Autodesk Inventor part; units mm, degrees
ref_plane "YZ Plane" through (0, 0, 0) normal (1, 0, 0) x (0, 1, 0)
ref_plane "XZ Plane" through (0, 0, 0) normal (0, 1, 0) x (-1, 0, 0)
ref_plane "XY Plane" through (0, 0, 0) normal (0, 0, 1) x (1, 0, 0)
sketch "Sketch1" plane through (0, 0, 0) normal (1, 0, 0) x (0, 1, 0)
  circle A0 centre (0, 0) radius 70
  line L0 (0, 0) -> (66.7602, 21.0494) construction
  line L1 (66.7602, -21.0494) -> (0, 0) construction
  line L2 (66.7602, -21.0494) -> (66.7602, 21.0494) construction
  circle A1 centre (66.7602, 21.0494) radius 1.65
  circle A2 centre (66.7602, -21.0494) radius 1.65
  circle A3 centre (0, 0) radius 57.5
  line L3 (64.3545, 28.6791) -> (-26.6041, 0)
  line L4 (-26.6041, 0) -> (64.3545, -28.6791)
  line L5 (74.7602, -21.0494) -> (74.7602, 21.0494)
  arc A4 (74.7602, 21.0494) -> (64.3545, 28.6791) centre (66.7602, 21.0494) ccw
  arc A5 (64.3545, -28.6791) -> (74.7602, -21.0494) centre (66.7602, -21.0494) ccw
  circle A6 centre (0, 0) radius 64.5
  point P0 (66.7602, 0)
  point P1 (51.8997, 24.7522)
  point P2 (51.8997, -24.7522)
  point P3 (58.6341, 26.8755)
  point P4 (58.6341, -26.8755)
  dimension "d0" = 140
  dimension "d1" = 35
  dimension "d2" = 3.3
  dimension "d3" = 3.3
  dimension "d4" = 115
  dimension "d5" = 8
  dimension "d6" = 8
  dimension "d7" = 7
extrude "Extrusion1" add sketch "Sketch1" against normal blind 7 contours A0 A2 L4 A6 L3 A1 | A0 A1 L3 A4 L5 A5 L4 A2 | A6 L4 A3 L3 picked at (61.9464, 3.0696)
extrude "Extrusion2" add sketch "Sketch1" along normal blind 20 contours A6 L4 A3 L3 picked at (61.9464, 3.0696)
fillet "Fillet1" radius 2 4 edges at (6.5, 51.8997, 24.7522) (6.5, 51.8997, -24.7522) (10, 58.6341, 26.8755) (10, 58.6341, -26.8755)
properties part number "ACOMPLE_PLASTICO" material "Steel, Mild, Welded"
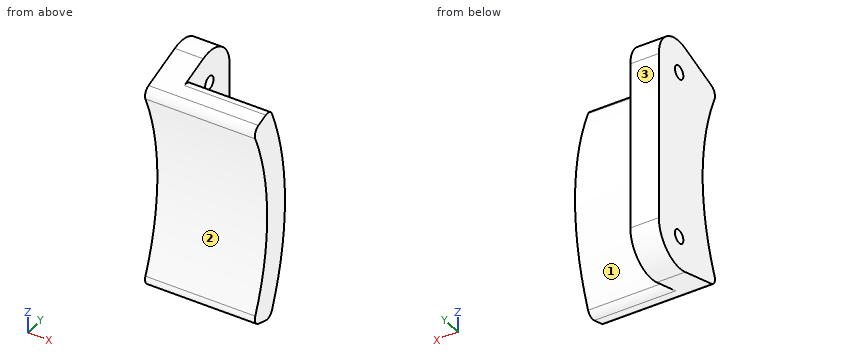
Can you work these out from the model? Positions are in its coordinate system, mm. Face numbers are marked on the shaded views. Round coordinates to 2 decimals unless told otherwise and drop trailing zeros. Order: outer loops, then holes, each group sorted by start corner. A loop starts at its lowest first (then second) coordinate and runs counter-clockwise, first axis right, second up. Notation, with made-up numbers: (-32.75, 2) - (-24.75, 2) arc R23 cw to (-24.75, 36) - close; hole circle Ø8 at (74, -30.75). An arc over 180 degrees is marked (long way). Answer in a Markdown table with one row per item.
(1) Suppose I cut it at B-B, the plane y = 55. Please give me the cut outline in (x, z).
From the geometry:
| item | result |
|---|---|
| outline | (-7, -25.73) - (20, -25.73) - (20, -16.77) - (-7, -16.77) - close; (-7, 16.77) - (20, 16.77) - (20, 25.73) - (-7, 25.73) - close |
(2) Suppose I cut it at C-C, the plane y = 62.25. Please give me the cut outline in (x, z), plus the area to 3 significant figures.
From the geometry:
| item | result |
|---|---|
| outline | (-7, -28.02) - (0, -28.02) - (0, -16.89) - (20, -16.89) - (20, 16.89) - (0, 16.89) - (0, 28.02) - (-7, 28.02) - close |
| area | 1,070 mm2 |
(3) For P1, Ø3, axis at x = 8, z = 14, coming from the -Y side; P2, Ø2, axis at x = 5, z = 13.5, coming from the +Y side; P3, Ø4, axis at x = 0, y = 72, coming from the -Z side, each with a flat end and sliding along its axis, tell me the tip position at first contact or that it passes through.
From the geometry:
| item | result |
|---|---|
| P1 | stops at y = 55.37 |
| P2 | stops at y = 63.28 |
| P3 | stops at z = -28.36 |
(4) If we mould it in two halves opening along Z, with no side actions, what happens to the marked faces 1, 2 and 3? For each: released by +Z, released by -Z, zero draft, split by the parting line, or undercut.
From the geometry:
| item | result |
|---|---|
| face 1 | split by the parting line |
| face 2 | undercut |
| face 3 | zero draft |
(5) Suppose I cut it at A-A, the plane x = -1.75. Please give me the cut outline in (y, z).
From the geometry:
| item | result |
|---|---|
| outline | (52.82, -22.73) arc R2 ccw to (54.05, -25.43) - (64.35, -28.68) arc R8 ccw to (74.76, -21.05) - (74.76, 21.05) arc R8 ccw to (64.35, 28.68) - (54.05, 25.43) arc R2 ccw to (52.82, 22.73) arc R57.5 cw to start; hole circle Ø3.3 at (66.76, -21.05); hole circle Ø3.3 at (66.76, 21.05) |
(6) Please list where these lines run through material, in increasing order: L1, parallel to X at y = 72, z = 5; L2, parallel to Y at x = -6, z = -0.5; L3, parallel to Z at x = -1.75, y = 63.5. Write a range as from..to.
From the geometry:
| item | result |
|---|---|
| L1 | x = -7..0 |
| L2 | y = 57.5..74.76 |
| L3 | z = -28.41..28.41 |
(7) Suppose I cut it at D-D, the plane z = 11.5. Please give me the cut outline in (x, y), plus the area to 3 significant figures.
From the geometry:
| item | result |
|---|---|
| outline | (-7, 56.34) - (20, 56.34) - (20, 63.47) - (0, 63.47) - (0, 74.76) - (-7, 74.76) - close |
| area | 272 mm2 |
